Input: dimensioned drawing with shaded views. Units: mm. Origin: part minimum x, y, z. A direction names the side the tool comes from. Give positions to 0.01 mm unless a question says otherwise; leave off trailing zeros. Write each loop counter-clockwise with the first axis right and the second up, starting at its lowest first coordinate (ties: lowest second). Pieces come first, ordered by that corner, then holes. Notation, with made-up numbers: (57, 59.5) - (84, 59.5) arc R31 ccw to (84, 84.5) - close; hole circle Ø5 at (45, 9.5). An arc over 180 degrees is marked (long way). Answer as CSV lines item,"result".
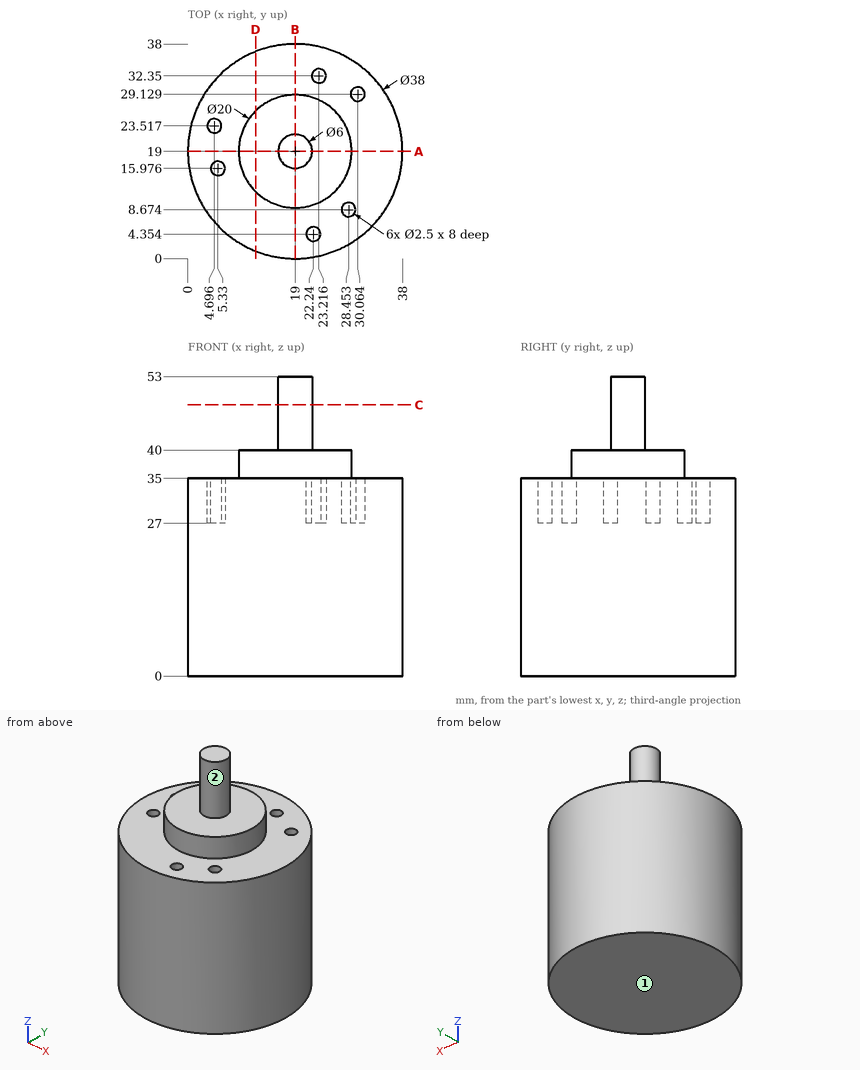
Item 1: Reachability of the marked faces 1 and 2 from +Z, -Z, +X, -X, +Y, -Y: full face, straight path, thin tool, end or side. Return the list, or none.
The answers:
face 1,"-Z, +X, -X, +Y, -Y"
face 2,"+Z"
Item 2: Cut plane C-C on z = 48. Return the cut outline in (x, y).
The answers:
outline,"circle Ø6 at (19, 19)"
Item 3: Ray query, line 1 (Z direction, x = 30, y = 10); line 2 (Z direction, x = 22.5, y = 5); line 3 (Y direction, x = 18.5, z = 23). Return the intervals inside material, ascending. Write a range as from..to.
The answers:
line 1,"0..35"
line 2,"0..27"
line 3,"0.01..37.99"
Item 4: Cut plane D-D on x = 12. Return the cut outline in (y, z), plus the area to 3 significant figures.
The answers:
outline,"(1.34, 0) - (36.66, 0) - (36.66, 35) - (26.14, 35) - (26.14, 40) - (11.86, 40) - (11.86, 35) - (1.34, 35) - close"
area,"1,310 mm²"
Item 5: Cut plane A-A on y = 19. Return the cut outline in (x, z), plus the area to 3 significant figures.
The answers:
outline,"(0, 0) - (38, 0) - (38, 35) - (29, 35) - (29, 40) - (22, 40) - (22, 53) - (16, 53) - (16, 40) - (9, 40) - (9, 35) - (0, 35) - close"
area,"1,510 mm²"
Item 6: Contact query for flat-ended pins moving along their axis: pin 1 (0.8 mm diameter, centred on x = 5, y = 16.5, fed in from +Z); pin 2 (1.5 mm diameter, centred on x = 16, z = 11, fed in from +Y); pin 3 (3 mm diameter, centred on x = 4.7, y = 23.52, fed in from +Z); pin 4 (3 mm diameter, centred on x = 20.5, y = 8.5, fed in from -Z). Output: stop coordinate, or through.
The answers:
pin 1,"z = 27"
pin 2,"y = 37.87"
pin 3,"z = 35"
pin 4,"z = 0"
